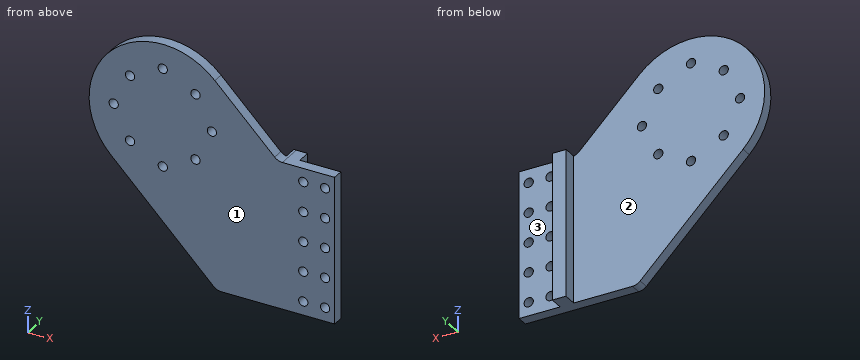
Autodesk Inventor part; units mm, degrees
ref_plane "YZ Plane" through (0, 0, 0) normal (1, 0, 0) x (0, 1, 0)
ref_plane "XZ Plane" through (0, 0, 0) normal (0, 1, 0) x (-1, 0, 0)
ref_plane "XY Plane" through (0, 0, 0) normal (0, 0, 1) x (1, 0, 0)
sketch "Skizze1" plane through (0, 0, 0) normal (0, 1, 0) x (-1, 0, 0)
  line L0 (0, 27) -> (0, -27)
  line L1 (0, 27) -> (20.8162, 27)
  line L2 (20.8162, 27) -> (43.9081, 50.0919)
  line L3 (0, -27) -> (43.1838, -27)
  line L4 (43.1838, -27) -> (82.0919, 11.9081)
  arc A0 (82.0919, 11.9081) -> (43.9081, 50.0919) centre (63, 31) ccw
  point P0 (0, 0)
  point P1 (0, 0)
  dimension "d43" = 54
  dimension "d44" = 135
  dimension "d46" = 31
  dimension "d47" = 63
  dimension "d48" = 54
extrude "Extrusion1" add sketch "Skizze1" along normal blind 4
sketch "Skizze5" plane through (0, 4, 0) normal (0, 1, 0) x (1, 0, 0)
  line L0 (0, -27) -> (0, 27)
  line L1 (0, 27) -> (-43.1838, 27)
  line L2 (-43.1838, 27) -> (-82.0919, -11.9081)
  arc A0 (-82.0919, -11.9081) -> (-43.9081, -50.0919) centre (-63, -31) ccw
  line L3 (-43.9081, -50.0919) -> (-20.8162, -27)
  line L4 (-20.8162, -27) -> (0, -27)
  line L5 (-20, -27) -> (-15, -27)
  line L6 (-15, -27) -> (-15, 27)
  line L7 (-15, 27) -> (-20, 27)
  line L8 (-20, 27) -> (-20, -27)
  dimension "d49" = 5
  dimension "d50" = 15
extrude "Extrusion4" add sketch "Skizze5" along normal blind 5 contours L4 L8 L1 L6
sketch "Skizze6" plane through (0, 4, 0) normal (0, 1, 0) x (1, 0, 0)
  point P0 (0, 0)
  point P1 (-3.5, 0)
  dimension "d51" = 3.5
hole "Bohrung1" at (-3.5, 4, 0) direction (0, -1, 0) diameter 3.4 end through all
pattern_linear "Rechteckige Anordnung1" count 5 spacing 11 along (0, 0, -1) count 2 spacing 8 along (-1, 0, 0) of "Bohrung1" first direction both ways yes
sketch "Skizze7" plane through (0, 0, 0) normal (0, -1, 0) x (1, 0, 0)
  line L0 (-51, 43) -> (-75, 43)
  line L1 (-75, 43) -> (-75, 19)
  line L2 (-75, 19) -> (-51, 19)
  line L3 (-51, 19) -> (-51, 43)
  line L4 (-51, 43) -> (-75, 19) construction
  line L5 (-63, 63.2011) -> (-63, 8.0055) construction
  circle A0 centre (-63, 31) radius 18
  line L6 (-63, 26.0548) -> (-63, -18.8231) construction
  line L7 (-38.3888, 31) -> (-81.0377, 31) construction
  arc A1 (-43.9081, 50.0919) -> (-82.0919, 11.9081) centre (-63, 31) ccw
  line L8 (-51, 19) -> (-75, 43) construction
  point P0 (-63, 13)
  point P1 (-81, 31)
  point P2 (-63, 13)
  point P3 (-63, 31)
  point P4 (-45, 31)
  point P5 (-63, 49)
  dimension "d32" = 24
  dimension "d33" = 24
  dimension "d35" = 36
hole "Bohrung2" at (-63, 0, 13) at (-81, 0, 31) at (-51, 0, 19) at (-75, 0, 19) at (-75, 0, 43) at (-51, 0, 43) at (-63, 0, 49) at (-45, 0, 31) direction (0, 1, 0) diameter 3.4 end through all
fillet "Rundung1" radius 4 2 edges at (-43.1838, 2, -27) (-20.8162, 2, 27)
equation "\"d48\" = d43"
properties part number "dynamixel_pro_frame_part3" material "Aluminium 6061"
Check sheet for the modelled part. Datum: model origin and axes. Units: mm. Face numbers are marked on the shaded views. A direction names the side the tool comes from. Round coordinates to 2 decimals unless told otherwise and drop trailing zeros. Loops run counter-clockwise (first coordinate to the right, second up) from the corner with the lowest first, then second, coordinate; pieces in that order, holes last.
1. Gauge pin test, flat ends, axial feed: pin 1 Ø5 at (y, z) = (2, -9.5) entering from -X; pin 2 Ø2 at (x, z) = (-45, 31) entering from +Y; pin 3 Ø4 at (y, z) = (5.5, -3) entering from -X; pin 4 Ø5 at (x, y) = (-44.5, 1.5) entering from +Z. Record the tip position at first contact, or that the pin passes through.
2. Scan lines: probe 1 along Z at (x, y) = (-63, 3.1); probe 2 along Z at (x, y) = (-52, 3.25); probe 3 along X at (y, z) = (3.1, 22). Record each from-to range of solid material in increasing order.
3. Sectioned sample at C-C on x = -51. Record the boundary of the cut face in (y, z).
4. Sectioned sample at B-B on z = 19. Record the boundary of the cut face in (x, y).
5. Sectioned sample at A-A on y = 2. Give the number of separate pieces and of enclosed holes in the cut face, and give its area (3 significant figures).
6. Set-up check for the marked faces 1, 2 and 3: record each of +Z, -Z, +X, -X, +Y, -Y from which the full face is reachable in a straight line by a thin tool's end or side.
7. Sectioned sample at D-D on z = 49. Record the boundary of the cut face in (x, y), and give its area (3 significant figures).
Recorded:
1. pin 1: stops at x = -63.18
1. pin 2: passes through
1. pin 3: stops at x = -68.51
1. pin 4: stops at z = 52.75
2. probe 1: z = -7.18 to 11.3, 14.7 to 47.3, 50.7 to 58
2. probe 2: z = -18.18 to 17.63, 20.37 to 41.63, 44.37 to 55.66
2. probe 3: x = -88.46 to -13.2, -9.8 to -5.2, -1.8 to 0
3. outline: (0, -19.18) - (4, -19.18) - (4, 17.3) - (0, 17.3) - close; (0, 20.7) - (4, 20.7) - (4, 41.3) - (0, 41.3) - close; (0, 44.7) - (4, 44.7) - (4, 55.19) - (0, 55.19) - close
4. outline: (-87.19, 0) - (-76.7, 0) - (-76.7, 4) - (-87.19, 4) - close; (-73.3, 0) - (-52.7, 0) - (-52.7, 4) - (-73.3, 4) - close; (-49.3, 0) - (0, 0) - (0, 4) - (-15, 4) - (-15, 9) - (-20, 9) - (-20, 4) - (-49.3, 4) - close
5. separate pieces: 1
5. enclosed holes: 18
5. area: 5,080 mm2
6. face 1: +Z, -Z, +X, -X, -Y
6. face 2: +Z, -Z, -X, +Y
6. face 3: +Z, -Z, +X, +Y
7. outline: (-83.12, 0) - (-64.7, 0) - (-64.7, 4) - (-83.12, 4) - close; (-61.3, 0) - (-42.82, 0) - (-42.82, 4) - (-61.3, 4) - close
7. area: 148 mm2
